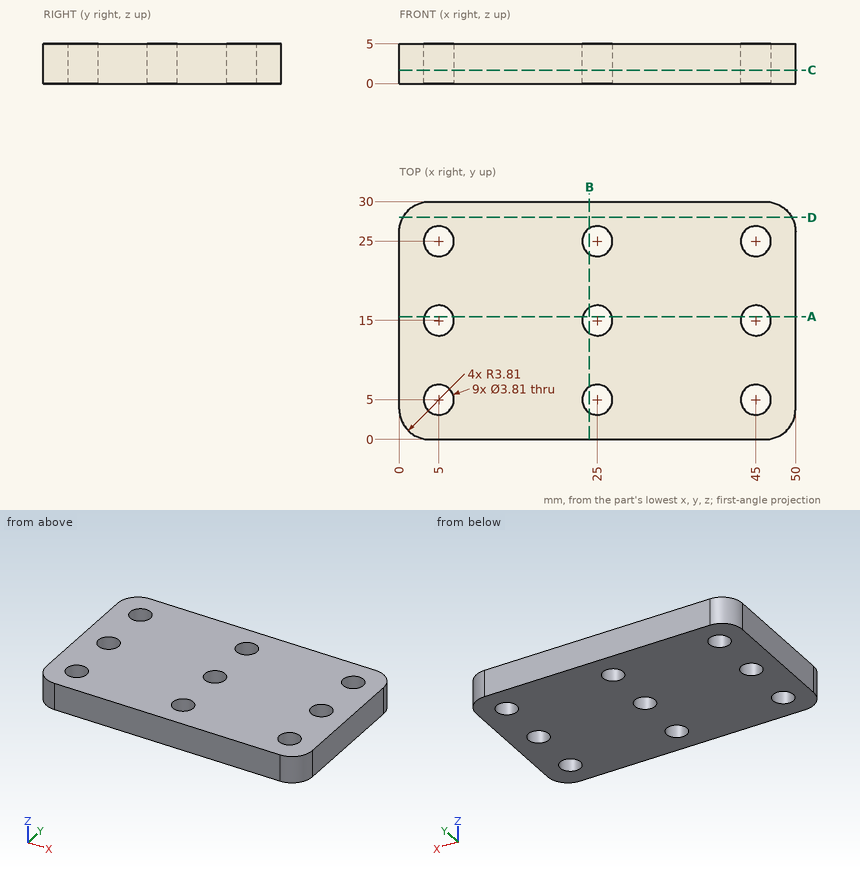
Study the drawing (mm; zero at the part's minimum x, y, z) and answer. Coordinates: 2 decimals unless noted, no trailing zeros. Write each loop counter-clockwise with the first axis right and the second up, starting at its lowest first coordinate (ties: lowest second). Pieces come first, ordered by that corner, then holes. Notation, with made-up numbers: M 16.5,19 L 27.5,19 A20 ccw 27.5,40 Z; hole C 60.5,17 d1. An arc over 180 degrees is marked long. Use one line per item in the form item = value.
Item 1: Find section D-D, the plane y = 28. Give the vertices of the cut face in (x, z), plus the area to 3 significant figures.
Model answer:
outline = M 0.46,0 L 49.54,0 L 49.54,5 L 0.46,5 Z
area = 245 mm2
Item 2: Find section C-C, the plane z = 1.7. Give the number of separate pieces and of enclosed holes in the cut face, plus the area to 3 significant figures.
Model answer:
separate_pieces = 1
enclosed_holes = 9
area = 1,380 mm2
Item 3: Find the intervals of material crossed by probe 1 along X at (y, z) = (16.5, 4.45) (1 decimal); probe 2 along X at (y, z) = (3.75, 1.7); probe 3 along Y at (x, z) = (4, 2), in increasing order.
Model answer:
probe_1 = 0 to 3.8, 6.2 to 23.8, 26.2 to 43.8, 46.2 to 50
probe_2 = 0 to 3.56, 6.44 to 23.56, 26.44 to 43.56, 46.44 to 50
probe_3 = 0 to 3.38, 6.62 to 13.38, 16.62 to 23.38, 26.62 to 30
Item 4: Find section A-A, the plane y = 15.5. Give the vertices of the cut face in (x, z), plus the area to 3 significant figures.
Model answer:
outline = M 0,0 L 3.16,0 L 3.16,5 L 0,5 Z; M 6.84,0 L 23.16,0 L 23.16,5 L 6.84,5 Z; M 26.84,0 L 43.16,0 L 43.16,5 L 26.84,5 Z; M 46.84,0 L 50,0 L 50,5 L 46.84,5 Z
area = 195 mm2
Item 5: Find section B-B, the plane x = 24. Give the vertices of the cut face in (y, z), plus the area to 3 significant figures.
Model answer:
outline = M 0,0 L 3.38,0 L 3.38,5 L 0,5 Z; M 6.62,0 L 13.38,0 L 13.38,5 L 6.62,5 Z; M 16.62,0 L 23.38,0 L 23.38,5 L 16.62,5 Z; M 26.62,0 L 30,0 L 30,5 L 26.62,5 Z
area = 101 mm2
